Work out the finished part from the listing and answer in its coordinate system (mm). Face numbers are marked on the shaded views. Coordinates: 2 decimals unless noted, no trailing zeros. Write each loop counter-clockwise with the first axis right and the second up, starting at its lowest first coordinate (ties: lowest second). Pieces come first, ordered by that corner, then holes. Notation, with made-up numbers: (54.5, 67.5) - (104.5, 67.5) arc R8 cw to (104.5, 73.5) - close; hole circle Ø11 at (6.5, 53). An arc over 180 degrees is marked (long way). Use a Markdown table: item, result. Add a question column.
(1) The part is cut by section B-B, the plane y = 39. Give the vertices of the cut face in (x, z), then the cut area to 3 significant figures.
(2) For a pull along X with two mould halves and no side action, classify the marked faces 1, 2 and 3 as released by +X, released by -X, zero draft, split by the parting line, or undercut.
(3) Given pin 1 Ø1 at (x, z) = (19, 17.5) entering from +Y; pin 2 Ø1 at (x, z) = (21, -27) entering from +Y; pin 3 Ø9 at (x, y) = (-23.57, 15.5) entering from +Z, each flat-ended and moving along its own axis, determine where each tip first touches the part or whether it passes through.
(4) The part is cut by section C-C, the plane x = -23.57. Give the vertices of the cut face in (y, z).
(5) Find the intervals of material crossed by line 1 (Y direction, x = -23.57, z = -32.4); line 2 (X direction, y = 15, z = -33); line 3 (Y direction, x = 22, z = -29.5), in increasing order. Write a range as from..to.
(6) The part is cut by section D-D, the plane x = -2. Give the vertices of the cut face in (y, z), then the cut area to 3 significant figures.
(7) The part is cut by section A-A, the plane z = 16.5. Give the vertices of the cut face in (x, y).
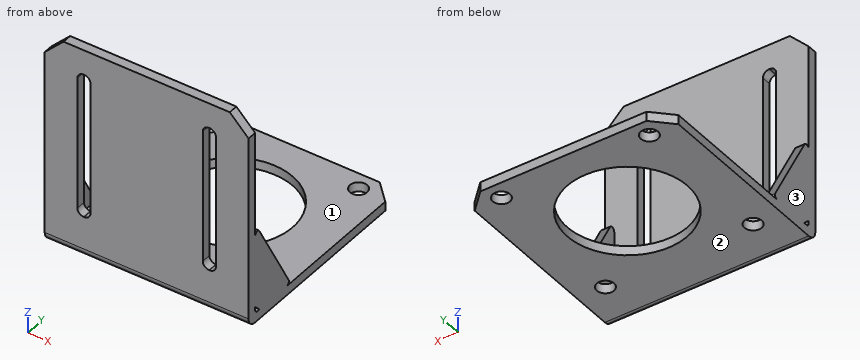
from build123d import *

# Parameters (mm, degrees)
SKETCH_1_W          = 65
SKETCH_1_H          = 65
EXTRUDE_1_DEPTH     = 3
SKETCH_1_3_W        = 65
SKETCH_1_3_H        = 3
EXTRUDE_2_DEPTH     = 68
CHAMFER_1_SIZE      = 6
CUT_EXTRUDE_1_REACH = 103.51
SKETCH_3_R          = 19.15
SKETCH_3_R_2        = 2.75
FILLET_1_R          = 3
FILLET_2_R          = 1
EXTRUDE_3_DEPTH     = 3
EXTRUDE_START       = -65
EXTRUDE_4_DEPTH     = 3


with BuildPart() as part:
    # Эскиз1 → Бобышка-Вытянуть1 (new body)
    with BuildSketch(Plane(origin=(0, 0, 0), x_dir=(1, 0, 0), z_dir=(0, 1, 0))):
        with Locations((0, -1.5)):
            Rectangle(SKETCH_1_W, SKETCH_1_H)
        with BuildLine():
            Line((-20.1, 20.5), (-19.9, 20.5))
            ThreePointArc((-19.9, 20.5), (-18.485786438, 19.914213562), (-17.9, 18.5))
            Line((-17.9, 18.5), (-17.9, -24))
            ThreePointArc((-17.9, -24), (-18.485786438, -25.414213562), (-19.9, -26))
            Line((-19.9, -26), (-20.1, -26))
            ThreePointArc((-20.1, -26), (-21.514213562, -25.414213562), (-22.1, -24))
            Line((-22.1, -24), (-22.1, 18.5))
            ThreePointArc((-22.1, 18.5), (-21.514213562, 19.914213562), (-20.1, 20.5))
        make_face(mode=Mode.SUBTRACT)
        with BuildLine():
            ThreePointArc((20.1, 20.5), (21.514213562, 19.914213562), (22.1, 18.5))
            Line((22.1, 18.5), (22.1, -24))
            ThreePointArc((22.1, -24), (21.514213562, -25.414213562), (20.1, -26))
            Line((20.1, -26), (19.9, -26))
            ThreePointArc((19.9, -26), (18.485786438, -25.414213562), (17.9, -24))
            Line((17.9, -24), (17.9, 18.5))
            ThreePointArc((17.9, 18.5), (18.485786438, 19.914213562), (19.9, 20.5))
            Line((19.9, 20.5), (20.1, 20.5))
        make_face(mode=Mode.SUBTRACT)
    extrude(amount=EXTRUDE_1_DEPTH)

    # Эскиз1<3> → Бобышка-Вытянуть2 (add)
    with BuildSketch(Plane(origin=(0, 0, 0), x_dir=(1, 0, 0), z_dir=(0, 1, 0))):
        with Locations((0, 32.5)):
            Rectangle(SKETCH_1_3_W, SKETCH_1_3_H)
    extrude(amount=EXTRUDE_2_DEPTH)

    # Фаска1
    chamfer_1_edges = [part.edges().sort_by_distance(p)[0] for p in [
        (32.5, 68, -32.5),
        (-32.5, 68, -32.5),
        (32.5, 1.5, 34),
        (-32.5, 1.5, 34),
    ]]
    chamfer(chamfer_1_edges, length=CHAMFER_1_SIZE)

    # Эскиз3 → Вырез-Вытянуть1 (cut, up to next)
    with BuildSketch(Plane(origin=(0, 0, -34), x_dir=(-1, 0, 0), z_dir=(0, 0, -1)), mode=Mode.PRIVATE) as cut_extrude_1_sk1:
        with Locations((0, 39)):
            Circle(SKETCH_3_R)
    cut_extrude_1_tool1 = extrude(cut_extrude_1_sk1.sketch, amount=-CUT_EXTRUDE_1_REACH, mode=Mode.PRIVATE) & part.part
    # Эскиз3 → Вырез-Вытянуть1 (cut, up to next)
    with BuildSketch(Plane(origin=(0, 0, -34), x_dir=(-1, 0, 0), z_dir=(0, 0, -1)), mode=Mode.PRIVATE) as cut_extrude_1_sk2:
        with Locations((-23.57, 62.57)):
            Circle(SKETCH_3_R_2)
    cut_extrude_1_tool2 = extrude(cut_extrude_1_sk2.sketch, amount=-CUT_EXTRUDE_1_REACH, mode=Mode.PRIVATE) & part.part
    # Эскиз3 → Вырез-Вытянуть1 (cut, up to next)
    with BuildSketch(Plane(origin=(0, 0, -34), x_dir=(-1, 0, 0), z_dir=(0, 0, -1)), mode=Mode.PRIVATE) as cut_extrude_1_sk3:
        with Locations((23.57, 62.5)):
            Circle(SKETCH_3_R_2)
    cut_extrude_1_tool3 = extrude(cut_extrude_1_sk3.sketch, amount=-CUT_EXTRUDE_1_REACH, mode=Mode.PRIVATE) & part.part
    # Эскиз3 → Вырез-Вытянуть1 (cut, up to next)
    with BuildSketch(Plane(origin=(0, 0, -34), x_dir=(-1, 0, 0), z_dir=(0, 0, -1)), mode=Mode.PRIVATE) as cut_extrude_1_sk4:
        with Locations((23.57, 15.5)):
            Circle(SKETCH_3_R_2)
    cut_extrude_1_tool4 = extrude(cut_extrude_1_sk4.sketch, amount=-CUT_EXTRUDE_1_REACH, mode=Mode.PRIVATE) & part.part
    # Эскиз3 → Вырез-Вытянуть1 (cut, up to next)
    with BuildSketch(Plane(origin=(0, 0, -34), x_dir=(-1, 0, 0), z_dir=(0, 0, -1)), mode=Mode.PRIVATE) as cut_extrude_1_sk5:
        with Locations((-23.57, 15.43)):
            Circle(SKETCH_3_R_2)
    cut_extrude_1_tool5 = extrude(cut_extrude_1_sk5.sketch, amount=-CUT_EXTRUDE_1_REACH, mode=Mode.PRIVATE) & part.part
    add(cut_extrude_1_tool1.solids().sort_by_distance((0, 39, -34))[0], mode=Mode.SUBTRACT)
    add(cut_extrude_1_tool2.solids().sort_by_distance((23.57, 62.57, -34))[0], mode=Mode.SUBTRACT)
    add(cut_extrude_1_tool3.solids().sort_by_distance((-23.57, 62.5, -34))[0], mode=Mode.SUBTRACT)
    add(cut_extrude_1_tool4.solids().sort_by_distance((-23.57, 15.5, -34))[0], mode=Mode.SUBTRACT)
    add(cut_extrude_1_tool5.solids().sort_by_distance((23.57, 15.43, -34))[0], mode=Mode.SUBTRACT)

    # Скругление1
    fillet_1_edges = [part.edges().sort_by_distance(p)[0] for p in [
        (0, 0, -34),
    ]]
    fillet(fillet_1_edges, radius=FILLET_1_R)

    # Скругление2
    fillet_2_edges = [part.edges().sort_by_distance(p)[0] for p in [
        (0, 3, -31),
    ]]
    fillet(fillet_2_edges, radius=FILLET_2_R)

    # Эскиз5 → Бобышка-Вытянуть3 (add)
    with BuildSketch(Plane.ZY.offset(32.5)):
        with BuildLine():
            Line((-31, 5), (-31, 17.312374786))
            ThreePointArc((-31, 17.312374786), (-30.509774395, 18.172682908), (-29.519739868, 18.189500891))
            Line((-29.519739868, 18.189500891), (-5.206600655, 4.877126106))
            ThreePointArc((-5.206600655, 4.877126106), (-4.718066148, 3.752135224), (-5.686860788, 3))
            Line((-5.686860788, 3), (-29, 3))
            Line((-29, 3), (-31, 5))
        make_face()
    extrude(amount=-EXTRUDE_3_DEPTH)

    # Эскиз5<2> → Бобышка-Вытянуть4 (add)
    with BuildSketch(Plane.ZY.offset(32.5).offset(EXTRUDE_START)):
        with BuildLine():
            Line((-31, 5), (-31, 17.312374786))
            ThreePointArc((-31, 17.312374786), (-30.509774395, 18.172682908), (-29.519739868, 18.189500891))
            Line((-29.519739868, 18.189500891), (-5.206600655, 4.877126106))
            ThreePointArc((-5.206600655, 4.877126106), (-4.718066148, 3.752135224), (-5.686860788, 3))
            Line((-5.686860788, 3), (-29, 3))
            Line((-29, 3), (-31, 5))
        make_face()
    extrude(amount=EXTRUDE_4_DEPTH)


solid = part.part
Model answer:
| question | item | result |
|---|---|---|
| 1 | outline | (-32.5, -34) - (-19.15, -34) - (-19.15, -31) - (-32.5, -31) - close; (19.15, -34) - (32.5, -34) - (32.5, -31) - (19.15, -31) - close |
| 1 | area | 80.1 mm^2 |
| 2 | face 1 | undercut |
| 2 | face 2 | zero draft |
| 2 | face 3 | released by -X |
| 3 | pin 1 | through |
| 3 | pin 2 | y = 3 |
| 3 | pin 3 | z = -31 |
| 4 | outline | (0, -31) arc R3 ccw to (3, -34) - (12.75, -34) - (12.75, -31) - (4, -31) arc R1 cw to (3, -30) - (3, 34) - (0, 34) - close; (18.25, -34) - (59.75, -34) - (59.75, -31) - (18.25, -31) - close; (65.25, -34) - (68, -34) - (68, -31) - (65.25, -31) - close |
| 5 | line 1 | 0.35..12.75, 18.25..59.75, 65.25..68 |
| 5 | line 2 | -32.5..-26.27, -20.87..20.85, 26.29..32.5 |
| 5 | line 3 | 0..3 |
| 6 | outline | (0, -31) arc R3 ccw to (3, -34) - (19.95, -34) - (19.95, -31) - (4, -31) arc R1 cw to (3, -30) - (3, 34) - (0, 34) - close; (58.05, -34) - (68, -34) - (68, -31) - (58.05, -31) - close |
| 6 | area | 283 mm^2 |
| 7 | outline | (-32.5, 0) - (-22.1, 0) - (-22.1, 3) - (-32.5, 3) - close; (-17.9, 0) - (17.9, 0) - (17.9, 3) - (-17.9, 3) - close; (22.1, 0) - (32.5, 0) - (32.5, 3) - (22.1, 3) - close |
